The listing builds one solid part. Answer for the finished solid, in the listing's coordinates (mm). A direction names the side the tool comes from. Round coordinates to 2 decimals unless told otherwise and drop trailing zeros. Order: outer loops, then holes, each group sorted by start corner. A loop starts at its lowest first (then second) coordinate and runs counter-clockwise, first axis right, second up. Notation, with made-up numbers: (51, 13.5) - (102, 13.5) arc R22 ccw to (102, 38.5) - close; hole circle Ø4 at (-22, 81.25). An arc over 180 degrees is marked (long way). One line per item, written item: value. Start each with the question number.
1. Section B-B, the plane x = 13.65 is taken. Give the vertices of the cut face in (y, z), then the cut area to 3 significant figures.
2. A tool of negligible diameter and unlimited length cuts with its end or side. For faces 5 (the flat face through (15, -10, 55.6)), 6 (the cylindrical face through (14.09, -11.38, 53.43)), from which of +Z, -Z, +X, -X, +Y, -Y can it reach the whole face along a straight path? Write none if from no direction.
3. Flat-ended cylindrical pins translate along their axes: P1, Ø2, axis at x = 15.5, z = 51, coming from the +Y side; P2, Ø1, axis at x = 14.5, z = 54.5, coming from the +Y side; P3, Ø0.9, axis at x = 15, z = 53, coming from the +Y side. Find the tip coordinate at first contact, or state that the pin passes through.
4. Section D-D, the plane y = -9.75 is taken. Give the vertices of the cut face in (x, z), then the cut area to 3 significant figures.
5. For a pull along Z with two mould halves and no side action, classify faces 1 (the flat face through (15, -12.3, 53)), 2 (the cylindrical face through (13.58, -8.74, 52.18)), 3 (the flat face through (15, -10, 49.5)), 4 (the flat face through (18.25, -12, 53)) as released by +Z, released by -Z, zero draft, split by the parting line, or undercut.
6. Section A-A, the plane y = -11.5 is taken. Give the vertices of the cut face in (x, z), then the cut area to 3 significant figures.
7. Section C-C, the plane z = 53.75 is taken. Give the vertices of the cut face in (x, y).
8. Straight lines are drawn through the part: line 1 (Z direction, x = 15.24, y = -10.8); line 2 (X direction, y = -11.6, z = 52.55); line 3 (X direction, y = -7.65, z = 52.55). For each, find the intervals that lie inside material, in ascending order.
from build123d import *

# Parameters (mm, degrees)
SKETCH1_W           = 5.5
SKETCH1_H           = 6.1
BOSS_EXTRUDE1_DEPTH = 1
BOSS_EXTRUDE2_REACH = 60.527
SKETCH2_W           = 5.5
SKETCH2_H           = 6.1
SKETCH2_R           = 1.45
SKETCH3_R           = 1.7
CUT_EXTRUDE1_DEPTH  = 5


with BuildPart() as part:
    # Sketch1 → Boss-Extrude1 (new body)
    with BuildSketch(Plane(origin=(0, -13.3, 0), x_dir=(1, 0, 0), z_dir=(0, 1, 0))):
        with Locations((15.5, -52.55)):
            Rectangle(SKETCH1_W, SKETCH1_H)
    extrude(amount=BOSS_EXTRUDE1_DEPTH)

    # Boss-Extrude2: up to this plane
    boss_extrude2_end = Plane(origin=(18.287867966, -10.962132034, -41.256060161), z_dir=(0.7071067811865521, 0.707106781186543, 0))
    # Sketch2 → Boss-Extrude2 (add, up to the surface)
    with BuildSketch(Plane(origin=(0, -12.3, 0), x_dir=(1, 0, 0), z_dir=(0, 1, 0)), mode=Mode.PRIVATE) as boss_extrude2_sk1:
        with Locations((15.5, -52.55)):
            Rectangle(SKETCH2_W, SKETCH2_H)
        with Locations((15.24, -52.55)):
            Circle(SKETCH2_R, mode=Mode.SUBTRACT)
    boss_extrude2_tool1 = split(extrude(boss_extrude2_sk1.sketch, amount=BOSS_EXTRUDE2_REACH, mode=Mode.PRIVATE), bisect_by=boss_extrude2_end, keep=Keep.BOTH, mode=Mode.PRIVATE)
    add(boss_extrude2_tool1.solids().sort_by_distance((12.832134, -12.3, 52.55))[0])

    # Sketch3 → Cut-Extrude1 (cut)
    with BuildSketch(Plane(origin=(0, -5.424264069, 0), x_dir=(1, 0, 0), z_dir=(0, 1, 0))):
        with Locations(Location((15.24, -52.55, 0), (0, 0, 270))):
            Circle(SKETCH3_R)
    extrude(amount=-CUT_EXTRUDE1_DEPTH, mode=Mode.SUBTRACT)


solid = part.part
Answer list:
1. outline: (-13.3, 49.5) - (-6.32, 49.5) - (-6.32, 51.95) - (-10.42, 51.95) - (-10.42, 53.15) - (-6.32, 53.15) - (-6.32, 55.6) - (-13.3, 55.6) - close
1. area: 37.6 mm²
2. face 5: +Z, +X, -X, +Y, -Y
2. face 6: +Y
3. P1: stops at y = -7.17
3. P2: stops at y = -6.67
3. P3: stops at y = -12.3
4. outline: (12.75, 49.5) - (17.08, 49.5) - (17.08, 55.6) - (12.75, 55.6) - close; hole circle Ø3.4 at (15.24, 52.55)
4. area: 17.3 mm²
5. face 1: undercut
5. face 2: undercut
5. face 3: released by -Z
5. face 4: zero draft
6. outline: (12.75, 49.5) - (18.25, 49.5) - (18.25, 55.6) - (12.75, 55.6) - close; hole circle Ø2.9 at (15.24, 52.55)
6. area: 26.9 mm²
7. outline: (12.75, -13.3) - (18.25, -13.3) - (18.25, -10.92) - (16.44, -9.12) - (16.44, -10.42) - (16.05, -10.42) - (16.05, -12.3) - (14.43, -12.3) - (14.43, -10.42) - (14.04, -10.42) - (14.04, -6.71) - (12.75, -5.42) - close
8. line 1: z = 49.5 to 51.1, 54 to 55.6
8. line 2: x = 12.75 to 13.79, 16.69 to 18.25
8. line 3: x = 12.75 to 13.54
